Design review of the part built by this model. Coordinates are the model's own, in mm. A direction names the side the tool comes from. Coordinates: 2 decimals unless noted, no trailing zeros. Loops run counter-clockwise (first coordinate to the right, second up) from the corner with the lowest first, then second, coordinate; pieces in that order, holes last.
from build123d import *

# Parameters (mm, degrees)
F1_DEPTH  = 70
F4_DEPTH  = 50
F6_REACH  = 161.8626818177
F7_R      = 12.5
F8_DEPTH  = 92.1420161514
F9_R      = 15
F10_R     = 7.5
F11_DEPTH = 25
F12_R     = 20
F13_DEPTH = 25


with BuildPart() as f1:
    # F0 (on Top) → F1 (new body)
    with BuildSketch(Plane.XY):
        Polygon((0, -10), (0, 0), (-125, 0), (-125, -40), (-115, -40), (-115, -10), align=None)
    extrude(amount=F1_DEPTH)

    # F3 (on offset) → F4 (join)
    with BuildSketch(Plane.XY.offset(60)):
        Polygon((-115, 0), (-28.3974596216, 0), (-50.0480947162, 37.5), align=None)
    extrude(amount=-F4_DEPTH)

    f6_end = Plane(origin=(-53.4880513164, 0, 35), x_dir=(0, 0, 1), z_dir=(0, 1, 0))
    # F5 (on face) → F6 (cut, up to a plane its end follows)
    with BuildSketch(Plane(origin=(-28.75, 49.7964607176, 0), x_dir=(-0.8660254038, -0.5, 0), z_dir=(-0.5, 0.8660254038, 0))):
        with BuildLine():
            ThreePointArc((49.5929214352, 10), (24.5929214352, 35), (49.5929214352, 60))
            Line((49.5929214352, 60), (49.5929214352, 65.1633962989))
            Line((49.5929214352, 65.1633962989), (18.7135729939, 65.1633962989))
            Line((18.7135729939, 65.1633962989), (18.7135729939, 2.6539005339))
            Line((18.7135729939, 2.6539005339), (49.5929214352, 2.6539005339))
            Line((49.5929214352, 2.6539005339), (49.5929214352, 10))
        make_face()
    f6_long = extrude(amount=-F6_REACH, mode=Mode.PRIVATE)
    add(split(f6_long, bisect_by=f6_end, keep=Keep.TOP, mode=Mode.PRIVATE), mode=Mode.SUBTRACT)

    # F7 (on face) → F8 (cut, through all)
    with BuildSketch(Plane(origin=(-28.75, 49.7964607176, 0), x_dir=(-0.8660254038, -0.5, 0), z_dir=(-0.5, 0.8660254038, 0))):
        with Locations((49.5929214352, 35)):
            Circle(F7_R)
    extrude(amount=-F8_DEPTH, mode=Mode.SUBTRACT)

    # F9
    f9_edges = [f1.edges().sort_by_distance(p)[0] for p in [
        (0, -5, 70),
        (0, -5, 0),
    ]]
    fillet(f9_edges, radius=F9_R)

    # F10 (on face) → F11 (cut)
    with BuildSketch(Plane(origin=(0, 0, 0), x_dir=(-1, 0, 0), z_dir=(0, 1, 0))):
        with Locations((15, 15)):
            Circle(F10_R)
        with Locations((15, 55)):
            Circle(F10_R)
    extrude(amount=-F11_DEPTH, mode=Mode.SUBTRACT)

    # F12 (on face) → F13 (cut)
    with BuildSketch(Plane(origin=(-125, 0, 0), x_dir=(0, -1, 0), z_dir=(-1, 0, 0))):
        with Locations((40, 35)):
            Circle(F12_R)
    extrude(amount=-F13_DEPTH, mode=Mode.SUBTRACT)


solid = f1.part
Q1. The part is to be moulded in two halves that separate along Z. For faces 6 (the cylindrical face through (-4.28, -4.93, 65.49)), 7 (the cylindrical face through (-120, -20, 35)), 8 (the cylindrical face through (-13.37, -4.93, 47.68)), 9 (the flat face through (0, -5, 35)), say which applies: pulls with the +Z half, pulls with the -Z half, needs draft (parallel to the pull), parting line crosses it, or undercut.
Q2. Take a section at A-A, the plane z = 49.5. Write out the cut boundary in (x, y), then the cut area to 3 significant figures.
Q3. Machinability: for faces 1 (the flat face through (-80, 7, 10)), 2 (the flat face through (-48, 0, 11)), 3 (the flat face through (-115, -19, 35)), 4 (the flat face through (-82.5, -9.5, 70)), 5 (the flat face through (-89.286, 14.846, 35.35)), which of the approach directions +Z, -Z, +X, -X, +Y, -Y give a long, thin tool a straight path to every point of the face, cutting with its end or side? Answer none if there is none.
Q4. Clearance check with flat-ended pins moving along their axes: pin 1 Ø24 at (y, z) = (-26.5, 38.5) entering from +X; pin 2 Ø2 at (y, z) = (15, 47) entering from +X; pin 3 Ø2 at (x, z) = (-68, 38) entering from -Y. State where each tip first meets the part, or that it passes through.
Q5. For line 1 (X direction, y = -13, z = 7.5); line 2 (X direction, y = 1.5, z = 40.5); line 3 (Z direction, x = -17, y = -6), list the stretches that pass through material, from the lowest coordinate up.
Q6. Take a section at C-C, the plane x = -90.5. Write out the cut boundary in (y, z).
Q7. Take a section at D-D, the plane z = 26. Write out the cut boundary in (x, y).
Q8. Take a section at B-B, the plane y = -22.5. Write out the cut boundary in (x, z), then the cut area to 3 significant figures.
Entries:
1. face 6: pulls with the +Z half
1. face 7: undercut
1. face 8: undercut
1. face 9: needs draft
2. outline: (-125, -26.23) - (-115, -26.23) - (-115, -10) - (-20.1, -10) - (-20.1, 0) - (-33.75, 0) - (-54.06, 35.18) - (-115, 0) - (-125, 0) - close; (-9.9, -10) - (0, -10) - (0, 0) - (-9.9, 0) - close
2. area: 2,740 mm2
3. face 1: -Z, +X, -X, +Y
3. face 2: +Y
3. face 3: +Z, -Z, +X, -Y
3. face 4: +Z, +X, -X, +Y, -Y
3. face 5: +Z, -Z, -X, +Y
4. pin 1: stops at x = -115
4. pin 2: stops at x = -39.76
4. pin 3: stops at y = -10
5. line 1: x = -125 to -115
5. line 2: x = -112.4 to -71.09, -45.17 to -29.97
5. line 3: z = 0 to 7.77, 22.23 to 47.77, 62.23 to 70
6. outline: (-10, 0) - (0, 0) - (0, 10) - (14.15, 10) - (14.15, 60) - (0, 60) - (0, 70) - (-10, 70) - close
7. outline: (-125, -22.14) - (-115, -22.14) - (-115, -10) - (-61.51, -10) - (-79.21, 20.66) - (-115, 0) - (-125, 0) - close; (-64.19, 29.34) - (-41.47, -10) - (0, -10) - (0, 0) - (-30.33, 0) - (-51.5, 36.66) - close
8. outline: (-125, 0) - (-115, 0) - (-115, 25.32) - (-125, 25.32) - close; (-125, 44.68) - (-115, 44.68) - (-115, 70) - (-125, 70) - close
8. area: 506 mm2
